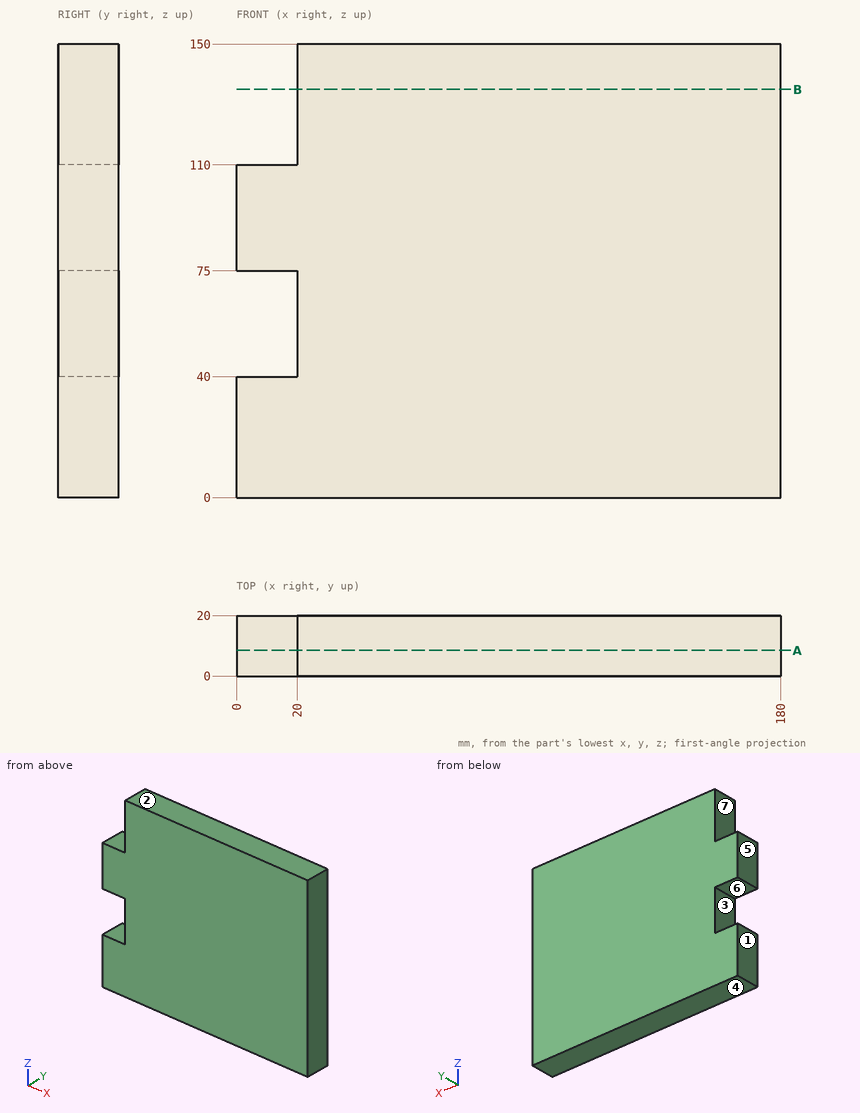
Answer from the drawing. Dimensions are ordinates in mm from the lowest x, y and z of the part. A direction names the side the tool comes from. Round coordinates to 2 decimals unless told otherwise and drop trailing zeros. Loops run counter-clockwise (first coordinate to the right, second up) from the corner with the lowest first, then second, coordinate; pieces in that order, holes last. Notation, with made-up numbers: (68.5, -17) - (86.5, -17) arc R21 ccw to (86.5, 19) - close; hole circle Ø5 at (73.25, 14). An arc over 180 degrees is marked (long way). One line per item, written item: value.
Q1. The mould has two halves that part along Z. Classify the marked faces 1, 2, 3 and 4: +Z half, -Z half, draft (parallel to the pull), parting line (faces both ways), or undercut.
Check values:
face 1: draft
face 2: +Z half
face 3: undercut
face 4: -Z half
Q2. Find section A-A on y = 8.5. Give the vertices of the cut face in (x, z), and give its area (3 significant figures).
Check values:
outline: (0, 0) - (180, 0) - (180, 150) - (20, 150) - (20, 110) - (0, 110) - (0, 75) - (20, 75) - (20, 40) - (0, 40) - close
area: 25,500 mm2
Q3. Each of these flat-tipped pins is pushed along its axis until it touches: pin 1 Ø10 at (y, z) = (5.5, 52.5) entering from -X; pin 2 Ø6 at (x, y) = (7.5, 6.5) entering from +Z. Where does it stop, or does it pass through?
Check values:
pin 1: x = 20
pin 2: z = 110
Q4. For the marked faces 5, 6 and 7, determine the directions among +Z, -Z, +X, -X, +Y, -Y from which every point of the face is accessible in a straight line to the end or side of a thin tool.
Check values:
face 5: +Z, -Z, -X, +Y, -Y
face 6: -X, +Y, -Y
face 7: +Z, -X, +Y, -Y
Q5. Find section B-B on z = 135. Give the vertices of the cut face in (x, y), and give its area (3 significant figures).
Check values:
outline: (20, 0) - (180, 0) - (180, 20) - (20, 20) - close
area: 3,200 mm2
Q6. A straight line is drawn through the part: probe 1 along X at (y, z) = (13.75, 60). Find the intervals that lie inside material, in ascending order.
Check values:
probe 1: 20 to 180
